```python
from build123d import *

# Parameters (mm, degrees)
SKETCH2_W           = 246
SKETCH2_H           = 251
BOSS_EXTRUDE1_DEPTH = 10
BOSS_EXTRUDE1_DRAFT = -2
SKETCH5_W           = 243
SKETCH5_H           = 248
CUT_EXTRUDE1_DEPTH  = 177.009232712
CUT_EXTRUDE1_DRAFT  = -2
CUT_EXTRUDE2_DEPTH  = 280.607703212


with BuildPart() as part:
    # Sketch2 → Boss-Extrude1 (with draft: the straight prism first)
    with BuildSketch(Plane(origin=(0, 0, 0), x_dir=(1, 0, 0), z_dir=(0, 1, 0))):
        Rectangle(SKETCH2_W, SKETCH2_H)
    extrude(amount=-BOSS_EXTRUDE1_DEPTH)
    # Boss-Extrude1: the draft: its side faces are tilted about the plane it starts from
    boss_extrude1_sides = [part.faces().sort_by_distance(p)[0] for p in [
        (0, -5, 125.5),
        (123, -5, 0),
        (0, -5, -125.5),
        (-123, -5, 0),
    ]]
    draft(boss_extrude1_sides, Plane(origin=(0, 0, 0), x_dir=(1, 0, 0), z_dir=(0, 1, 0)), BOSS_EXTRUDE1_DRAFT)


with BuildPart() as cut_extrude1_tool:
    # Sketch5 → Cut-Extrude1 (with draft: the straight prism first)
    with BuildSketch(Plane(origin=(0, 0, 0), x_dir=(1, 0, 0), z_dir=(0, 1, 0))):
        Rectangle(SKETCH5_W, SKETCH5_H)
    extrude(amount=-CUT_EXTRUDE1_DEPTH)
    # Cut-Extrude1: the draft: its side faces are tilted about the plane it starts from
    cut_extrude1_sides = [cut_extrude1_tool.faces().sort_by_distance(p)[0] for p in [
        (121.5, -88.504616356, 0),
        (0, -88.504616356, -124),
        (-121.5, -88.504616356, 0),
        (0, -88.504616356, 124),
    ]]
    draft(cut_extrude1_sides, Plane(origin=(0, 0, 0), x_dir=(1, 0, 0), z_dir=(0, 1, 0)), CUT_EXTRUDE1_DRAFT)


with BuildPart() as part_1:
    add(part.part)

    # Cut-Extrude1: cut by cut_extrude1_tool
    add(cut_extrude1_tool.part, mode=Mode.SUBTRACT)

    # Sketch9 → Cut-Extrude2 (cut, through all, along a direction that is not the sketch's normal)
    with BuildSketch(Plane(origin=(0, -4.377218727, 125.347144154), x_dir=(1, 0, 0), z_dir=(0, -0.03489949670250105, 0.9993908270190958))):
        Polygon((-122.651217373, -5.614028847), (-122.650792305, -5.626208607), (122.650792305, -5.626208607), (122.651217373, -5.614028847), align=None)
    extrude(amount=-CUT_EXTRUDE2_DEPTH, dir=(0, 0, 1), mode=Mode.SUBTRACT)


solid = part_1.part
```
Model file for the job. Use its own axes, mm. Coordinates: 2 decimals unless noted, no trailing zeros. Order: outer loops, then holes, each group sorted by start corner. A loop starts at its lowest first (then second) coordinate and runs counter-clockwise, first axis right, second up. Notation, with made-up numbers: (62.5, -7) -> (121.5, -7) arc R32 cw to (121.5, 20) -> close; hole circle Ø4 at (88.25, 77.25). An arc over 180 degrees is marked (long way). Return JSON: item names as keys, results as strings.
Item 1: Slice it at C-C (y = -7.25). Write the cut outline in (x, z).
Model answer:
{"outline": "(-122.75, -125.25) -> (122.75, -125.25) -> (122.75, 125.25) -> (-122.75, 125.25) -> close; hole (-121.25, -123.75) -> (121.25, -123.75) -> (121.25, 123.75) -> (-121.25, 123.75) -> close"}
Item 2: Pin check, flat tips, straight feed: P1, Ø4, axis at x = 16, y = -7.5, coming from the -Z side; P2, Ø4, axis at x = -24, y = -7, coming from the +Z side; P3, Ø4, axis at y = -2, z = -37, coming from the -X side; P4, Ø3, axis at y = -5, z = 81, coming from the +X side. Stop position of each tip, or through.
Model answer:
{"P1": "stops at z = -125.31", "P2": "stops at z = 125.33", "P3": "stops at x = -123", "P4": "stops at x = 122.88"}
Item 3: Slice it at B-B (x = -75.5). Write the cut outline in (y, z), then the cut area to 3 significant figures.
Model answer:
{"outline": "(-9.99, -125.15) -> (0, -125.5) -> (0, -124) -> (-9.99, -123.65) -> close; (-9.99, 123.65) -> (0, 124) -> (0, 125.5) -> (-9.99, 125.15) -> close", "area": "30.0 mm²"}
Item 4: Wall check: line 1 along X through (y, z) = (-1.75, 25.5); line 2 along Z through (x, y) = (-37.5, -1); line 3 along X through (y, z) = (-0.75, 23.5). Give the ranges that are in metal, low to high. Write a range as from..to.
Model answer:
{"line 1": "x = -122.94..-121.44, 121.44..122.94", "line 2": "z = -125.47..-123.97, 123.97..125.47", "line 3": "x = -122.97..-121.47, 121.47..122.97"}
Item 5: Slice it at A-A (z = 65). Write the cut outline in (x, y), then the cut area to 3 significant figures.
Model answer:
{"outline": "(-123, 0) -> (-122.65, -9.99) -> (-121.15, -9.99) -> (-121.5, 0) -> close; (121.15, -9.99) -> (122.65, -9.99) -> (123, 0) -> (121.5, 0) -> close", "area": "30.0 mm²"}
